The listing builds one solid part. Answer for the finished solid, in the listing's coordinates (mm). A direction names the side the tool comes from. Coordinates: 2 decimals unless noted, no trailing zeros. Loops run counter-clockwise (first coordinate to the right, second up) from the corner with the lowest first, then second, coordinate; pieces in that order, holes last. Notation, with made-up numbers: (27.5, -28.5) - (73.5, -28.5) arc R16 ccw to (73.5, -12.5) - close; hole circle Ø2 at (20, 13.5). An arc over 180 degrees is marked (long way). Put each result on its own line as item: value.
```python
from build123d import *

# Parameters (mm, degrees)
SKETCH1_R           = 4
SKETCH1_R_2         = 12
BOSS_EXTRUDE1_DEPTH = 2.5
FILLET1_R           = 4
CHAMFER1_SIZE       = 1


with BuildPart() as part:
    # Sketch1 → Boss-Extrude1 (new body, symmetric)
    with BuildSketch(Plane(origin=(0, 0, 0), x_dir=(1, 0, 0), z_dir=(0, 1, 0))):
        with BuildLine():
            Line((39.081081081, 10.801347209), (3.405405405, 17.674931797))
            ThreePointArc((3.405405405, 17.674931797), (0, 18), (-3.405405405, 17.674931797))
            Line((-3.405405405, 17.674931797), (-39.081081081, 10.801347209))
            ThreePointArc((-39.081081081, 10.801347209), (-48, 0), (-39.081081081, -10.801347209))
            Line((-39.081081081, -10.801347209), (-3.405405405, -17.674931797))
            ThreePointArc((-3.405405405, -17.674931797), (0, -18), (3.405405405, -17.674931797))
            Line((3.405405405, -17.674931797), (39.081081081, -10.801347209))
            ThreePointArc((39.081081081, -10.801347209), (48, 0), (39.081081081, 10.801347209))
        make_face()
        with Locations((37, 0)):
            Circle(SKETCH1_R, mode=Mode.SUBTRACT)
        with Locations((-37, 0)):
            Circle(SKETCH1_R, mode=Mode.SUBTRACT)
        Circle(SKETCH1_R_2, mode=Mode.SUBTRACT)
        with BuildLine():
            Line((-29.082089608, -7.635882073), (-14.68452203, -10.40984211))
            ThreePointArc((-14.68452203, -10.40984211), (-18, 0), (-14.68452203, 10.40984211))
            Line((-14.68452203, 10.40984211), (-29.082089608, 7.635882073))
            ThreePointArc((-29.082089608, 7.635882073), (-26, 0), (-29.082089608, -7.635882073))
        make_face(mode=Mode.SUBTRACT)
        with BuildLine():
            ThreePointArc((14.68452203, 10.40984211), (18, 0), (14.68452203, -10.40984211))
            Line((14.68452203, -10.40984211), (29.082089608, -7.635882073))
            ThreePointArc((29.082089608, -7.635882073), (26, 0), (29.082089608, 7.635882073))
            Line((29.082089608, 7.635882073), (14.68452203, 10.40984211))
        make_face(mode=Mode.SUBTRACT)
    extrude(amount=BOSS_EXTRUDE1_DEPTH, both=True)

    # Fillet1
    fillet1_edges = [part.edges().sort_by_distance(p)[0] for p in [
        (14.68452203, 0, 10.40984211),
        (29.082089608, 0, 7.635882073),
        (29.082089608, 0, -7.635882073),
        (14.68452203, 0, -10.40984211),
        (-14.68452203, 0, 10.40984211),
        (-14.68452203, 0, -10.40984211),
        (-29.082089608, 0, -7.635882073),
        (-29.082089608, 0, 7.635882073),
    ]]
    fillet(fillet1_edges, radius=FILLET1_R)

    # Chamfer1
    chamfer1_edges = [part.edges().sort_by_distance(p)[0] for p in [
        (33, 2.5, 0),
        (-41, 2.5, 0),
    ]]
    chamfer(chamfer1_edges, length=CHAMFER1_SIZE)


solid = part.part
```
1) The part is cut by section A-A (z = 0). Give the vertices of the cut face in (x, y), and give its area (3 significant figures).
Found:
outline: (-48, -2.5) - (-41, -2.5) - (-41, 1.5) - (-42, 2.5) - (-48, 2.5) - close; (-33, -2.5) - (-26, -2.5) - (-26, 2.5) - (-32, 2.5) - (-33, 1.5) - close; (-18, -2.5) - (-12, -2.5) - (-12, 2.5) - (-18, 2.5) - close; (12, -2.5) - (18, -2.5) - (18, 2.5) - (12, 2.5) - close; (26, -2.5) - (33, -2.5) - (33, 1.5) - (32, 2.5) - (26, 2.5) - close; (41, -2.5) - (48, -2.5) - (48, 2.5) - (42, 2.5) - (41, 1.5) - close
area: 198 mm^2
2) For a pull along X with two mould halves and no side action, classify faces 1 (the face through (26, 0, 0)), 2 (the face through (-21.49, 0.04, 14.19)), 3 (the face through (0, 0, 18)) as pulls with the +X half, pulls with the -X half, needs draft (parallel to the pull), parting line crosses it, or undercut.
Found:
face 1: undercut
face 2: pulls with the -X half
face 3: parting line crosses it
3) Each of these flat-tipped pins is pushed along its axis until it touches: pin 1 (1.5 mm diameter, centred on x = -23, y = -1, fed in from -Z); pin 2 (1 mm diameter, centred on x = 18.5, y = 0, fed in from -Z); pin 3 (1.5 mm diameter, centred on x = 37.5, y = 0, fed in from +Z); pin 4 (10.5 mm diameter, centred on x = -37, z = 0, fed in from -Y). Where does it stop, or does it pass through?
Found:
pin 1: stops at z = -14.04
pin 2: stops at z = -14.86
pin 3: stops at z = 11.25
pin 4: stops at y = -2.5
4) The part is cut by section B-B (y = 0.2). Give the vertices of the cut face in (x, z), and give its area (3 significant figures).
Found:
outline: (-39.08, -10.8) - (-3.41, -17.67) arc R18 ccw to (3.41, -17.67) - (39.08, -10.8) arc R11 ccw to (39.08, 10.8) - (3.41, 17.67) arc R18 ccw to (-3.41, 17.67) - (-39.08, 10.8) arc R11 ccw to start; hole circle Ø8 at (-37, 0); hole (-26.57, -3.5) arc R4 ccw to (-23.54, -8.7) - (-22.17, -8.97) arc R4 ccw to (-17.52, -4.12) arc R18 cw to (-17.52, 4.12) arc R4 ccw to (-22.17, 8.97) - (-23.54, 8.7) arc R4 ccw to (-26.57, 3.5) arc R11 cw to start; hole circle Ø24 at (0, 0); hole (17.52, -4.12) arc R4 ccw to (22.17, -8.97) - (23.54, -8.7) arc R4 ccw to (26.57, -3.5) arc R11 cw to (26.57, 3.5) arc R4 ccw to (23.54, 8.7) - (22.17, 8.97) arc R4 ccw to (17.52, 4.12) arc R18 cw to start; hole circle Ø8 at (37, 0)
area: 1,720 mm^2
5) For faces 4 (the face through (-20.994, 0.035, -14.286)), 5 (the face through (26.26, -0.04, 6.75)), determine the directions among +Z, -Z, +X, -X, +Y, -Y from which every point of the face is accessible in a straight line to the end or side of a thin tool.
Found:
face 4: -Z, -X, +Y, -Y
face 5: +Y, -Y
6) The part is cut by section C-C (x = 37). Give the vertices of the cut face in (y, z), and give its area (3 significant figures).
Found:
outline: (-2.5, -11.2) - (2.5, -11.2) - (2.5, -5) - (1.5, -4) - (-2.5, -4) - close; (-2.5, 4) - (1.5, 4) - (2.5, 5) - (2.5, 11.2) - (-2.5, 11.2) - close
area: 71.0 mm^2
7) Straight lines are drawn through the part: L1, parallel to X at y = -1.6, z = -2.5; L2, parallel to X at y = 1.15, z = 7.5; L3, parallel to X at y = 1.1, z = -6. For each, find the intervals that lie inside material, in ascending order. Write a range as [from, to].
Found:
L1: x = [-47.71, -40.12], [-33.88, -26.29], [-17.83, -11.74], [11.74, 17.83], [26.29, 33.88], [40.12, 47.71]
L2: x = [-45.05, -25.71], [-18.26, -9.37], [9.37, 18.26], [25.71, 45.05]
L3: x = [-46.22, -26.59], [-17.53, -10.39], [10.39, 17.53], [26.59, 46.22]
